Source: CAD feature listing. Evaluate the final solid. Frame: model axes, mm. A direction names the side the tool comes from. Round coordinates to 2 decimals unless told otherwise and drop trailing zeros. Write each loop counter-clockwise with the first axis right and the second up, starting at its lowest first coordinate (ties: lowest second). Pieces come first, ordered by that corner, then holes.
from build123d import *

# Parameters (mm, degrees)
F1_DEPTH = 20
F2_R     = 10


with BuildPart() as f1:
    # F0 (on Front) → F1 (new body)
    with BuildSketch(Plane.XZ):
        with BuildLine():
            Line((47.276331, 35.251416), (47.276331, 50.491416))
            Line((47.276331, 50.491416), (-67.023669, 50.491416))
            Line((-67.023669, 50.491416), (-67.023669, 35.852298))
            Line((-67.023669, 35.852298), (-19.011813, 19.254055))
            ThreePointArc((-19.011813, 19.254055), (-11.837012, 6.076339), (2.219168, 0.827168))
            Line((2.219168, 0.827168), (19.999168, 0.827168))
            Line((19.999168, 0.827168), (38.225762, -36.226879))
            Line((38.225762, -36.226879), (77.082462, -36.226879))
            Line((77.082462, -36.226879), (48.419438, 17.255383))
            Line((48.419438, 17.255383), (62.516331, 35.251416))
            Line((62.516331, 35.251416), (47.276331, 35.251416))
        make_face()
    extrude(amount=F1_DEPTH)

    # F2
    f2_edges = [f1.edges().sort_by_distance(p)[0] for p in [
        (47.276331, -10, 35.251416),
    ]]
    fillet(f2_edges, radius=F2_R)


solid = f1.part
1) Section query C-C on z = 12. Return the cut outline in (x, y), then the cut area to 3 significant figures.
Taken from the geometry:
outline: (-16.61, -20) - (51.24, -20) - (51.24, 0) - (-16.61, 0) - close
area: 1,360 mm2
2) Section query B-B on x = 18.5. Return the cut outline in (y, z).
Taken from the geometry:
outline: (-20, 0.83) - (0, 0.83) - (0, 50.49) - (-20, 50.49) - close
3) Section query A-A on y = -5.75. Return the cut outline in (x, z), then the cut area to 3 significant figures.
Taken from the geometry:
outline: (-67.02, 35.85) - (-19.01, 19.25) arc R21.44 ccw to (2.22, 0.83) - (20, 0.83) - (38.23, -36.23) - (77.08, -36.23) - (48.42, 17.26) - (62.52, 35.25) - (57.28, 35.25) arc R10 cw to (47.28, 45.25) - (47.28, 50.49) - (-67.02, 50.49) - close
area: 5,970 mm2
4) Reachability of faces 1 (the face through (55.37, -9.86, 26.13)), 2 (the face through (60, -10, 35.251)), 3 (the face through (11, -10, 0.827)) from +Z, -Z, +X, -X, +Y, -Y: full face, straight path, thin tool, end or side. Return the list, or none.
Taken from the geometry:
face 1: +X, +Y, -Y
face 2: +Z, +X, +Y, -Y
face 3: -Z, -X, +Y, -Y
5) Material intervals for line 1 (X direction, y = -12.75, z = 44.5); line 2 (Z direction, x = 1.5, y = -5); line 3 (Z direction, x = -22, y = -2), sorted ascending.
Taken from the geometry:
line 1: x = -67.02 to 47.3
line 2: z = 0.84 to 50.49
line 3: z = 20.29 to 50.49
6) Contact query for flat-ended pins moving along their axis: P1, Ø9, axis at x = 13.5, y = -11, coming from the -Z side; P2, Ø8, axis at y = -11.5, z = 34, coming from the +X side; P3, Ø1.5, axis at y = -17.5, z = -23.5, coming from the -X side. Output: stop coordinate, or through.
Taken from the geometry:
P1: stops at z = 0.83
P2: stops at x = 62.52
P3: stops at x = 31.6
